from build123d import *

# Parameters (mm, degrees)
EXTRUDE_1_DEPTH     = 3
EXTRUDE_1_2_DEPTH   = 3
EXTRUDE_1_3_DEPTH   = 3
SKETCH_2_R          = 35
EXTRUDE_1_4_DEPTH   = 3
SKETCH_3_R          = 35
EXTRUDE_2_DEPTH     = 1
SKETCH_4_R          = 1.505
CUT_EXTRUDE_1_DEPTH = 5


with BuildPart() as part:
    # Sketch 2 → Extrude 1 (new body)
    with BuildSketch(Plane(origin=(0, 0, 0), x_dir=(1, 0, 0), z_dir=(0, 1, 0))):
        with BuildLine():
            ThreePointArc((4.933437269, 11.253544382), (3.336493541, 10.122155344), (1.39173101, 9.902680687))
            ThreePointArc((1.39173101, 9.902680687), (-5.877852523, -8.090169944), (8.987940463, 4.383711468))
            ThreePointArc((8.987940463, 4.383711468), (8.595708593, 6.301111944), (9.178240759, 8.169514123))
            ThreePointArc((9.178240759, 8.169514123), (9.312956952, 8.786525533), (9.030558816, 9.351417404))
            ThreePointArc((9.030558816, 9.351417404), (7.64120828, 10.517220927), (6.103130316, 11.478318707))
            ThreePointArc((6.103130316, 11.478318707), (5.478620398, 11.572334106), (4.933437269, 11.253544382))
        make_face()
    extrude(amount=EXTRUDE_1_DEPTH)



with BuildPart() as body_2:
    # Sketch 2 → Extrude 1 2 (new body)
    with BuildSketch(Plane(origin=(0, 0, 0), x_dir=(1, 0, 0), z_dir=(0, 1, 0))):
        with BuildLine():
            ThreePointArc((-2.226769615, -15.8442891), (4.94427191, -15.216904261), (11.114533927, -11.509436805))
            ThreePointArc((11.114533927, -11.509436805), (14.127161486, -7.511545005), (15.756924048, -2.778370843))
            ThreePointArc((15.756924048, -2.778370843), (16.57293705, -0.458749656), (18.091681962, 1.475141128))
            ThreePointArc((18.091681962, 1.475141128), (18.635380141, 2.307784992), (18.711347307, 3.299315376))
            ThreePointArc((18.711347307, 3.299315376), (18.07007381, 5.871322893), (17.07708688, 8.329051789))
            ThreePointArc((17.07708688, 8.329051789), (16.432821214, 9.08656434), (15.503544365, 9.440609604))
            ThreePointArc((15.503544365, 9.440609604), (13.138141438, 10.112464253), (11.114533927, 11.509436805))
            ThreePointArc((11.114533927, 11.509436805), (4.94427191, 15.216904261), (-2.226769615, 15.8442891))
            ThreePointArc((-2.226769615, 15.8442891), (-4.685022346, 15.903561216), (-6.993579766, 16.750368343))
            ThreePointArc((-6.993579766, 16.750368343), (-7.953483115, 17.010154935), (-8.919959693, 16.776004264))
            ThreePointArc((-8.919959693, 16.776004264), (-11.167919794, 15.371322893), (-13.198509039, 13.667456206))
            ThreePointArc((-13.198509039, 13.667456206), (-13.719857247, 12.820638895), (-13.769411964, 11.827438089))
            ThreePointArc((-13.769411964, 11.827438089), (-13.677434002, 9.370191718), (-14.380704741, 7.013938349))
            ThreePointArc((-14.380704741, 7.013938349), (-16, 0), (-14.380704741, -7.013938349))
            ThreePointArc((-14.380704741, -7.013938349), (-13.677434002, -9.370191718), (-13.769411964, -11.827438089))
            ThreePointArc((-13.769411964, -11.827438089), (-13.719857247, -12.820638895), (-13.198509039, -13.667456206))
            ThreePointArc((-13.198509039, -13.667456206), (-11.167919794, -15.371322893), (-8.919959693, -16.776004264))
            ThreePointArc((-8.919959693, -16.776004264), (-7.953483115, -17.010154935), (-6.993579766, -16.750368343))
            ThreePointArc((-6.993579766, -16.750368343), (-4.685022346, -15.903561216), (-2.226769615, -15.8442891))
        make_face()
        with BuildLine():
            ThreePointArc((10.785528556, 5.260453761), (10.593186617, 6.200705058), (10.878847662, 7.116928659))
            ThreePointArc((10.878847662, 7.116928659), (11.297524269, 9.034502472), (10.419875557, 10.790097005))
            ThreePointArc((10.419875557, 10.790097005), (8.816778784, 12.135254916), (7.042073442, 13.244213893))
            ThreePointArc((7.042073442, 13.244213893), (5.101195454, 13.536398874), (3.40685257, 12.545650862))
            ThreePointArc((3.40685257, 12.545650862), (2.623746261, 11.990842401), (1.670077212, 11.883216825))
            ThreePointArc((1.670077212, 11.883216825), (-7.053423028, -9.708203932), (10.785528556, 5.260453761))
        make_face(mode=Mode.SUBTRACT)
    extrude(amount=EXTRUDE_1_2_DEPTH)


with BuildPart() as body_3:
    # Sketch 2 → Extrude 1 3 (new body)
    with BuildSketch(Plane(origin=(0, 0, 0), x_dir=(1, 0, 0), z_dir=(0, 1, 0))):
        with BuildLine():
            ThreePointArc((22.469851157, 10.95927867), (23.776412907, 7.725424859), (24.620193825, 4.341204442))
            ThreePointArc((24.620193825, 4.341204442), (24.516588458, 2.018942005), (23.437340957, -0.039907608))
            ThreePointArc((23.437340957, -0.039907608), (22.300880056, -1.81261067), (21.665770566, -3.820259909))
            ThreePointArc((21.665770566, -3.820259909), (20.923243358, -6.798373876), (19.773469019, -9.644165229))
            ThreePointArc((19.773469019, -9.644165229), (19.107216775, -11.641695573), (18.98466424, -13.743837434))
            ThreePointArc((18.98466424, -13.743837434), (18.647632371, -16.043847525), (17.366459261, -17.983495008))
            ThreePointArc((17.366459261, -17.983495008), (14.694631307, -20.225424859), (11.73678907, -22.073689821))
            ThreePointArc((11.73678907, -22.073689821), (9.496170427, -22.69277382), (7.204582268, -22.302567971))
            ThreePointArc((7.204582268, -22.302567971), (5.167455737, -21.769524797), (3.061808221, -21.785897512))
            ThreePointArc((3.061808221, -21.785897512), (0, -22), (-3.061808221, -21.785897512))
            ThreePointArc((-3.061808221, -21.785897512), (-5.167455737, -21.769524797), (-7.204582268, -22.302567971))
            ThreePointArc((-7.204582268, -22.302567971), (-9.496170427, -22.69277382), (-11.73678907, -22.073689821))
            ThreePointArc((-11.73678907, -22.073689821), (-14.694631307, -20.225424859), (-17.366459261, -17.983495008))
            ThreePointArc((-17.366459261, -17.983495008), (-18.647632371, -16.043847525), (-18.98466424, -13.743837434))
            ThreePointArc((-18.98466424, -13.743837434), (-19.107216775, -11.641695573), (-19.773469019, -9.644165229))
            ThreePointArc((-19.773469019, -9.644165229), (-20.923243358, -6.798373876), (-21.665770566, -3.820259909))
            ThreePointArc((-21.665770566, -3.820259909), (-22.300880056, -1.81261067), (-23.437340957, -0.039907608))
            ThreePointArc((-23.437340957, -0.039907608), (-24.516588458, 2.018942005), (-24.620193825, 4.341204442))
            ThreePointArc((-24.620193825, 4.341204442), (-14.694631307, 20.225424859), (3.479327524, 24.756701719))
            ThreePointArc((3.479327524, 24.756701719), (5.655914528, 23.9405486), (7.280491049, 22.277903712))
            ThreePointArc((7.280491049, 22.277903712), (8.615246116, 20.649269795), (10.328374381, 19.424847043))
            ThreePointArc((10.328374381, 19.424847043), (12.93127555, 17.798373876), (15.28248415, 15.825475607))
            ThreePointArc((15.28248415, 15.825475607), (16.976365134, 14.574561246), (18.937750033, 13.8084093))
            ThreePointArc((18.937750033, 13.8084093), (21.021041042, 12.777130739), (22.469851157, 10.95927867))
        make_face()
        with BuildLine():
            ThreePointArc((12.503850668, -12.948116406), (15.893056671, -8.45048813), (17.726539554, -3.125667198))
            ThreePointArc((17.726539554, -3.125667198), (18.326181707, -1.421107788), (19.442222095, 0))
            ThreePointArc((19.442222095, 0), (20.529100807, 1.664494981), (20.680962813, 3.646611731))
            ThreePointArc((20.680962813, 3.646611731), (19.972186842, 6.489356882), (18.874674972, 9.205794083))
            ThreePointArc((18.874674972, 9.205794083), (17.586757035, 10.72009797), (15.729088083, 11.427851419))
            ThreePointArc((15.729088083, 11.427851419), (13.990886243, 11.921559689), (12.503850668, 12.948116406))
            ThreePointArc((12.503850668, 12.948116406), (5.562305899, 17.119017293), (-2.505115817, 17.824825237))
            ThreePointArc((-2.505115817, 17.824825237), (-4.311547767, 17.868380988), (-6.007977036, 18.490652015))
            ThreePointArc((-6.007977036, 18.490652015), (-7.926869827, 19.00997786), (-9.858902819, 18.54189945))
            ThreePointArc((-9.858902819, 18.54189945), (-12.343490298, 16.989356882), (-14.58782578, 15.106135807))
            ThreePointArc((-14.58782578, 15.106135807), (-15.63002583, 13.413307424), (-15.729088083, 11.427851419))
            ThreePointArc((-15.729088083, 11.427851419), (-15.661498642, 9.622158987), (-16.178292833, 7.890680642))
            ThreePointArc((-16.178292833, 7.890680642), (-18, 0), (-16.178292833, -7.890680642))
            ThreePointArc((-16.178292833, -7.890680642), (-15.661498642, -9.622158987), (-15.729088083, -11.427851419))
            ThreePointArc((-15.729088083, -11.427851419), (-15.63002583, -13.413307424), (-14.58782578, -15.106135807))
            ThreePointArc((-14.58782578, -15.106135807), (-12.343490298, -16.989356882), (-9.858902819, -18.54189945))
            ThreePointArc((-9.858902819, -18.54189945), (-7.926869827, -19.00997786), (-6.007977036, -18.490652015))
            ThreePointArc((-6.007977036, -18.490652015), (-4.311547767, -17.868380988), (-2.505115817, -17.824825237))
            ThreePointArc((-2.505115817, -17.824825237), (5.562305899, -17.119017293), (12.503850668, -12.948116406))
        make_face(mode=Mode.SUBTRACT)
    extrude(amount=EXTRUDE_1_3_DEPTH)


with BuildPart() as body_4:
    # Sketch 2 → Extrude 1 4 (new body)
    with BuildSketch(Plane(origin=(0, 0, 0), x_dir=(1, 0, 0), z_dir=(0, 1, 0))):
        Circle(SKETCH_2_R)
        with BuildLine():
            ThreePointArc((-21.571057111, -10.520907523), (-21.071193566, -12.019578048), (-20.979247092, -13.596734588))
            ThreePointArc((-20.979247092, -13.596734588), (-20.516153338, -16.757030106), (-18.755776002, -19.422174609))
            ThreePointArc((-18.755776002, -19.422174609), (-15.870201812, -21.843458848), (-12.675732195, -23.839585007))
            ThreePointArc((-12.675732195, -23.839585007), (-9.597042635, -24.6902284), (-6.448319149, -24.15407171))
            ThreePointArc((-6.448319149, -24.15407171), (-4.919941122, -23.754149829), (-3.340154423, -23.76643365))
            ThreePointArc((-3.340154423, -23.76643365), (0, -24), (3.340154423, -23.76643365))
            ThreePointArc((3.340154423, -23.76643365), (4.919941122, -23.754149829), (6.448319149, -24.15407171))
            ThreePointArc((6.448319149, -24.15407171), (9.597042635, -24.6902284), (12.675732195, -23.839585007))
            ThreePointArc((12.675732195, -23.839585007), (15.870201812, -21.843458848), (18.755776002, -19.422174609))
            ThreePointArc((18.755776002, -19.422174609), (20.516153338, -16.757030106), (20.979247092, -13.596734588))
            ThreePointArc((20.979247092, -13.596734588), (21.071193566, -12.019578048), (21.571057111, -10.520907523))
            ThreePointArc((21.571057111, -10.520907523), (22.825356391, -7.416407865), (23.635386072, -4.167556264))
            ThreePointArc((23.635386072, -4.167556264), (24.111884402, -2.66129392), (24.964527497, -1.331302695))
            ThreePointArc((24.964527497, -1.331302695), (26.447451878, 1.497629765), (26.589809331, 4.688500797))
            ThreePointArc((26.589809331, 4.688500797), (25.67852594, 8.343458848), (24.26743925, 11.836020963))
            ThreePointArc((24.26743925, 11.836020963), (22.276722717, 14.333814244), (19.414206911, 15.750827598))
            ThreePointArc((19.414206911, 15.750827598), (17.942654929, 16.325642065), (16.671800891, 17.264155208))
            ThreePointArc((16.671800891, 17.264155208), (14.106846055, 19.416407865), (11.267317507, 21.190742229))
            ThreePointArc((11.267317507, 21.190742229), (9.982022971, 22.109379732), (8.980607357, 23.331281394))
            ThreePointArc((8.980607357, 23.331281394), (6.748381541, 25.615814497), (3.757673726, 26.737237856))
            ThreePointArc((3.757673726, 26.737237856), (-15.870201812, 21.843458848), (-26.589809331, 4.688500797))
            ThreePointArc((-26.589809331, 4.688500797), (-26.447451878, 1.497629765), (-24.964527497, -1.331302695))
            ThreePointArc((-24.964527497, -1.331302695), (-24.111884402, -2.66129392), (-23.635386072, -4.167556264))
            ThreePointArc((-23.635386072, -4.167556264), (-22.825356391, -7.416407865), (-21.571057111, -10.520907523))
        make_face(mode=Mode.SUBTRACT)
    extrude(amount=EXTRUDE_1_4_DEPTH)


with BuildPart() as part_1:
    add(part.part)

    add(body_2.part)  # Extrude 2 merges body 2

    add(body_3.part)  # Extrude 2 merges body 3

    add(body_4.part)  # Extrude 2 merges body 4
    # Sketch 3 → Extrude 2 (add)
    with BuildSketch(Plane.XZ):
        Circle(SKETCH_3_R)
    extrude(amount=EXTRUDE_2_DEPTH)

    # Sketch 4 → Cut-Extrude 1 (cut, through all)
    with BuildSketch(Plane(origin=(0, 3, 0), x_dir=(1, 0, 0), z_dir=(0, 1, 0))):
        Circle(SKETCH_4_R)
    extrude(amount=-CUT_EXTRUDE_1_DEPTH, mode=Mode.SUBTRACT)


solid = part_1.part
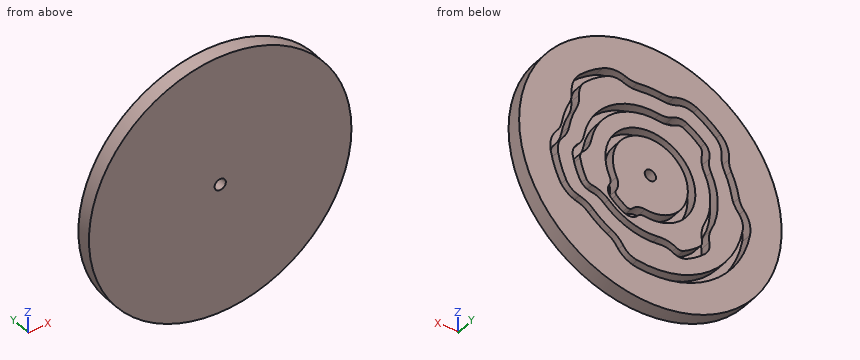
Geometry check sheet. Reference: the model listing, model coordinates, mm. Give positions to 0.01 mm unless a question says otherwise; leave off trailing zeros. Loops run counter-clockwise (first coordinate to the right, second up) from the corner with the lowest first, then second, coordinate; pieces in that order, holes last.
(1) Depth check by flat-ended pin: pin 1 Ø1.8 at (x, z) = (0, 0) entering from +Y; pin 2 Ø1.5 at (y, z) = (1, -14) entering from +X (3 decimals). Enter the tip coordinate at first touch or a pass-through.
From the geometry:
pin 1: passes through
pin 2: stops at x = 32.395
(2) Section check C-C on x = 28.5. Record the cut outline in (y, z), then the cut area to 3 significant figures.
From the geometry:
outline: (-1, -20.32) - (3, -20.32) - (3, 20.32) - (-1, 20.32) - close
area: 163 mm2
(3) Section check B-B on y = 1.1. Count the separate pieces of the cut face and the enclosed holes in it, then the cut area to 3 significant figures.
From the geometry:
separate pieces: 4
enclosed holes: 4
area: 3,140 mm2
(4) Thickness scan on L1, parallel to X at y = 0.8, z = -28; L2, parallel to Y at x = 17, z = 4; L3, parallel to Z at x = 25, y = 1.45. Record the ranges inside material, lowest first.
From the geometry:
L1: x = -21 to 21
L2: y = -1 to 0
L3: z = -24.49 to -10.2, 1.29 to 24.49
